Read the model definition and answer for the solid it produces. Units are mm, in the model's axes. A direction names the side the tool comes from. Give positions to 0.01 mm unless a question says otherwise; leave off trailing zeros. Loops run counter-clockwise (first coordinate to the right, second up) from the corner with the lowest first, then second, coordinate; pieces in that order, holes last. Notation, with made-up numbers: (70.25, 10.5) -> (122.25, 10.5) arc R18 ccw to (122.25, 26.5) -> close; hole circle Ø3 at (-7.75, 84). An arc over 180 degrees is marked (long way). Answer as CSV lines item,"result". Start each with the question number.
```python
from build123d import *

# Parameters (mm, degrees)
F0_R      = 2
F1_DEPTH  = 8
F3_DEPTH  = 185
F5_DEPTH  = 5
F6_R      = 2.5
F7_DEPTH  = 5
F8_R      = 2.012254
F9_DEPTH  = 3
F10_R     = 4
F10_R_2   = 2
F11_DEPTH = 4
F13_DEPTH = 340
F15_DEPTH = 320
F16_R     = 1.5
F17_DEPTH = 25


with BuildPart() as f1:
    # F0 (on Top) → F1 (new body)
    with BuildSketch(Plane.XY):
        Polygon((248.954639, 211.431908), (-84.845372, 211.431908), (-84.845372, -69.567305), (248.954639, -69.567305), (248.954639, -32.408092), align=None)
        with Locations((-44.415361, -24.153092)):
            Circle(F0_R, mode=Mode.SUBTRACT)
        with BuildLine():
            Line((-54.415363, 33.177276), (-54.415363, -42.732489))
            ThreePointArc((-54.415363, -42.732489), (-60.347495, -48.664621), (-66.279627, -42.732489))
            Line((-66.279627, -42.732489), (-66.279627, 33.177276))
            ThreePointArc((-66.279627, 33.177276), (-60.347495, 39.109408), (-54.415363, 33.177276))
        make_face(mode=Mode.SUBTRACT)
        with BuildLine():
            Line((-19.355729, -34.152674), (54.985007, -34.152674))
            ThreePointArc((54.985007, -34.152674), (63.564824, -42.732488), (54.98501, -51.312305))
            Line((54.98501, -51.312305), (-19.355726, -51.312305))
            ThreePointArc((-19.355726, -51.312305), (-27.935546, -42.732491), (-19.355729, -34.152674))
        make_face(mode=Mode.SUBTRACT)
        with Locations((80.044639, -24.153092)):
            Circle(F0_R, mode=Mode.SUBTRACT)
        with Locations((-44.415361, 48.236908)):
            Circle(F0_R, mode=Mode.SUBTRACT)
        with BuildLine():
            ThreePointArc((-34.415361, 23.177276), (-30.004497, 33.826044), (-19.355729, 38.236908))
            Line((-19.355729, 38.236908), (54.985007, 38.236908))
            ThreePointArc((54.985007, 38.236908), (65.633775, 33.826044), (70.044639, 23.177276))
            Line((70.044639, 23.177276), (70.044639, 0.90654))
            ThreePointArc((70.044639, 0.90654), (65.633775, -9.742228), (54.985007, -14.153092))
            Line((54.985007, -14.153092), (-19.355729, -14.153092))
            ThreePointArc((-19.355729, -14.153092), (-30.004497, -9.742228), (-34.415361, 0.90654))
            Line((-34.415361, 0.90654), (-34.415361, 23.177276))
        make_face(mode=Mode.SUBTRACT)
        with Locations((80.044639, 48.236908)):
            Circle(F0_R, mode=Mode.SUBTRACT)
        with BuildLine():
            ThreePointArc((212.465007, -34.152674), (221.044824, -42.732488), (212.46501, -51.312305))
            Line((212.46501, -51.312305), (105.104274, -51.312305))
            ThreePointArc((105.104274, -51.312305), (96.524457, -42.732491), (105.104271, -34.152674))
            Line((105.104271, -34.152674), (212.465007, -34.152674))
        make_face(mode=Mode.SUBTRACT)
        with Locations((237.524639, -24.153092)):
            Circle(F0_R, mode=Mode.SUBTRACT)
        with BuildLine():
            Line((90.044639, 0.90654), (90.044639, 23.177276))
            ThreePointArc((90.044639, 23.177276), (94.455503, 33.826044), (105.104271, 38.236908))
            Line((105.104271, 38.236908), (212.465007, 38.236908))
            ThreePointArc((212.465007, 38.236908), (223.113775, 33.826044), (227.524639, 23.177276))
            Line((227.524639, 23.177276), (227.524639, 0.90654))
            ThreePointArc((227.524639, 0.90654), (223.113775, -9.742228), (212.465007, -14.153092))
            Line((212.465007, -14.153092), (105.104271, -14.153092))
            ThreePointArc((105.104271, -14.153092), (94.455503, -9.742228), (90.044639, 0.90654))
        make_face(mode=Mode.SUBTRACT)
        with Locations((237.524639, 48.236908)):
            Circle(F0_R, mode=Mode.SUBTRACT)
        with BuildLine():
            Line((-54.415363, 180.316908), (-54.415363, 63.29654))
            ThreePointArc((-54.415363, 63.29654), (-60.347495, 57.364408), (-66.279627, 63.29654))
            Line((-66.279627, 63.29654), (-66.279627, 180.316908))
            ThreePointArc((-66.279627, 180.316908), (-60.347495, 186.24904), (-54.415363, 180.316908))
        make_face(mode=Mode.SUBTRACT)
        with BuildLine():
            Line((-34.415361, 73.29654), (-34.415361, 178.117276))
            ThreePointArc((-34.415361, 178.117276), (-30.004497, 188.766044), (-19.355729, 193.176908))
            Line((-19.355729, 193.176908), (54.985007, 193.176908))
            ThreePointArc((54.985007, 193.176908), (65.633775, 188.766044), (70.044639, 178.117276))
            Line((70.044639, 178.117276), (70.044639, 73.29654))
            ThreePointArc((70.044639, 73.29654), (65.633775, 62.647772), (54.985007, 58.236908))
            Line((54.985007, 58.236908), (-19.355729, 58.236908))
            ThreePointArc((-19.355729, 58.236908), (-30.004497, 62.647772), (-34.415361, 73.29654))
        make_face(mode=Mode.SUBTRACT)
        with Locations((-44.415361, 203.176908)):
            Circle(F0_R, mode=Mode.SUBTRACT)
        with Locations((80.044639, 203.176908)):
            Circle(F0_R, mode=Mode.SUBTRACT)
        with BuildLine():
            ThreePointArc((227.524639, 73.29654), (223.113775, 62.647772), (212.465007, 58.236908))
            Line((212.465007, 58.236908), (105.104271, 58.236908))
            ThreePointArc((105.104271, 58.236908), (94.455503, 62.647772), (90.044639, 73.29654))
            Line((90.044639, 73.29654), (90.044639, 178.117276))
            ThreePointArc((90.044639, 178.117276), (94.455503, 188.766044), (105.104271, 193.176908))
            Line((105.104271, 193.176908), (212.465007, 193.176908))
            Line((212.465007, 193.176908), (212.465007, 170.316908))
            ThreePointArc((212.465007, 170.316908), (223.113775, 165.906044), (227.524639, 155.257276))
            Line((227.524639, 155.257276), (227.524639, 73.29654))
        make_face(mode=Mode.SUBTRACT)
        with Locations((237.524639, 180.316908)):
            Circle(F0_R, mode=Mode.SUBTRACT)
    extrude(amount=F1_DEPTH)

    # F2 (on face) → F3 (join)
    with BuildSketch(Plane.XY.offset(8)):
        Polygon((15.154628, 211.431908), (-84.845372, 211.431908), (-84.845372, 71.431908), (-81.845372, 71.431908), (-81.845372, 208.431908), (15.154628, 208.431908), align=None)
    extrude(amount=F3_DEPTH)

    # F4 (on face) → F5 (cut)
    with BuildSketch(Plane(origin=(-84.845372, 0, 0), x_dir=(0, -1, 0), z_dir=(-1, 0, 0))):
        Polygon((-169.016169, 40), (-201.431908, 143.553324), (-201.431908, 40), align=None)
        Polygon((-71.431908, 193), (-206.431908, 193), (-158.537665, 40), (-71.431908, 40), align=None)
    extrude(amount=-F5_DEPTH, mode=Mode.SUBTRACT)

    # F6 (on face) → F7 (cut)
    with BuildSketch(Plane(origin=(0, 211.431908, 0), x_dir=(-1, 0, 0), z_dir=(0, 1, 0))):
        Polygon((12.845372, 83.034229), (12.845372, 55.132884), (75.345372, 55.132884), (75.345372, 148.132884), (67.845372, 148.132884), (67.845372, 178.132884), (2.845372, 178.132884), (1.345372, 83.215967), align=None)
        with Locations((11.345372, 185.632884)):
            Circle(F6_R)
        with Locations((1.345372, 185.632884)):
            Circle(F6_R)
        with Locations((75.345372, 161.632884)):
            Circle(F6_R)
        with Locations((75.345372, 185.632884)):
            Circle(F6_R)
        with Locations((75.345372, 47.632884)):
            Circle(F6_R)
        with Locations((65.345372, 47.632884)):
            Circle(F6_R)
        with Locations((1.345372, 47.632884)):
            Circle(F6_R)
        with Locations((1.345372, 71.632884)):
            Circle(F6_R)
    extrude(amount=-F7_DEPTH, mode=Mode.SUBTRACT)

    # F8 (on face) → F9 (join)
    with BuildSketch(Plane.XY.offset(40)):
        Polygon((14.154628, 208.488166), (-81.845372, 208.488166), (-81.845372, 201.431908), (-81.845372, 169.016169), (-81.845372, 71.523808), align=None)
        Polygon((-71.845372, 103.213636), (-71.845372, 198.488166), (-5.066284, 198.488166), align=None, mode=Mode.SUBTRACT)
        with Locations((-44.408604, 203.142822)):
            Circle(F8_R, mode=Mode.SUBTRACT)
    extrude(amount=-F9_DEPTH)

    # F10 (on face) → F11 (join)
    with BuildSketch(Plane.XY.offset(8)):
        with Locations((237.524639, 48.236908)):
            Circle(F10_R)
        with Locations((237.524639, 48.236908)):
            Circle(F10_R_2, mode=Mode.SUBTRACT)
        with Locations((237.524639, -24.153092)):
            Circle(F10_R)
        with Locations((237.524639, -24.153092)):
            Circle(F10_R_2, mode=Mode.SUBTRACT)
        with Locations((80.044639, 48.236908)):
            Circle(F10_R)
        with Locations((80.044639, 48.236908)):
            Circle(F10_R_2, mode=Mode.SUBTRACT)
        with Locations((80.044639, -24.153092)):
            Circle(F10_R)
        with Locations((80.044639, -24.153092)):
            Circle(F10_R_2, mode=Mode.SUBTRACT)
    extrude(amount=F11_DEPTH)

    # F12 (on face) → F13 (cut)
    with BuildSketch(Plane.YZ.offset(248.954639)):
        Polygon((57.743425, 4), (37.743425, 4), (37.743425, 0), (211.431908, 0), (211.431908, 8), (57.743425, 8), align=None)
    extrude(amount=-F13_DEPTH, mode=Mode.SUBTRACT)

    # F14 (on face) → F15 (cut)
    with BuildSketch(Plane(origin=(0, 211.431908, 0), x_dir=(-1, 0, 0), z_dir=(0, 1, 0))):
        Polygon((-69.711687, 8), (-69.711687, 4), (-89.711687, 4), (-89.711687, 0), (-20.75227, 0), (93.97424, 0), (93.97424, 17.639369), (93.97424, 194.899216), (-20.75227, 194.899216), (-20.75227, 10.883192), align=None)
    extrude(amount=-F15_DEPTH, mode=Mode.SUBTRACT)

    # F16 (on face) → F17 (cut)
    with BuildSketch(Plane.XY.offset(8)):
        with Locations((214.26287, -63.217305)):
            Circle(F16_R)
        with Locations((112.66287, -63.217305)):
            Circle(F16_R)
        with Locations((172.65287, -63.217305)):
            Circle(F16_R)
    extrude(amount=-F17_DEPTH, mode=Mode.SUBTRACT)


solid = f1.part
```
(1) Each of these flat-tipped pins is pushed along its axis until it touches: P1, Ø6, axis at x = 229.5, y = -37, coming from the +Z side; P2, Ø1.2, axis at x = 228, z = 1.5, coming from the +Y side; P3, Ø4.5, axis at y = -17.5, z = 1.5, coming from the -X side. Where does it stop, or does it pass through?
(2) Find section D-D on x = 223. Write down the section's boundary in (y, z), then the cut area to 3 significant figures.
(3) Find the intervals of material crossed by line 1 along Y through (x, z) = (129, 5.25); line 2 along X through (y, z) = (21, 3.5); line 3 along X through (y, z) = (-63.5, 5.5), in increasing order. Write a range as from..to.
(4) Find section B-B on x = 194. Write down the section's boundary in (y, z), then the cut area to 3 significant figures.
(5) The mould has two halves that part along Y. Classify faces 4 (the face through (239.2, 46.5, 12)), 5 (the face through (235.527, 48.325, 7.944)): pulls with the +Y half, pulls with the -Y half, needs draft (parallel to the pull), parting line crosses it, or undercut.
(6) Find section C-C on z = 2. Write down the section's boundary in (x, y) (3 decimals), then the cut area to 3 significant figures.
(7) A tool of negligible diameter and unlimited length cuts with its end or side. For faces 1 (the face through (94.34, 33.71, 3.94)), 2 (the face through (238, -22, 12)), 3 (the face through (241.34, 49.44, 9.97)), from which of +Z, -Z, +X, -X, +Y, -Y can it reach the whole face along a straight path? Write none if from no direction.
(8) Find section A-A on y = 21. Write down the section's boundary in (x, z).
Answer block:
1,P1,"stops at z = 8"
1,P2,"stops at y = 37.74"
1,P3,"stops at x = 89.71"
2,outline,"(-69.57, 0) -> (-9.85, 0) -> (-9.85, 8) -> (-69.57, 8) -> close; (33.94, 0) -> (37.74, 0) -> (37.74, 4) -> (57.74, 4) -> (57.74, 8) -> (33.94, 8) -> close"
2,area,"588 mm2"
3,line 1,"y = -69.57..-51.31, -34.15..-14.15, 38.24..57.74"
3,line 2,"x = 89.71..90.04, 227.52..248.95"
3,line 3,"x = 69.71..111.19, 114.14..171.18, 174.13..212.79, 215.74..248.95"
4,outline,"(-69.57, 0) -> (-51.31, 0) -> (-51.31, 8) -> (-69.57, 8) -> close; (-34.15, 0) -> (-14.15, 0) -> (-14.15, 8) -> (-34.15, 8) -> close; (38.24, 4) -> (57.74, 4) -> (57.74, 8) -> (38.24, 8) -> close"
4,area,"384 mm2"
5,face 4,"needs draft"
5,face 5,"undercut"
6,outline,"(89.712, -69.567) -> (248.955, -69.567) -> (248.955, 37.743) -> (216.289, 37.743) arc R15.06 cw to (227.525, 23.177) -> (227.525, 0.907) arc R15.06 cw to (212.465, -14.153) -> (105.104, -14.153) arc R15.06 cw to (90.045, 0.907) -> (90.045, 23.177) arc R15.06 cw to (101.281, 37.743) -> (89.712, 37.743) -> close; hole (105.104, -51.312) -> (212.465, -51.312) arc R8.58 ccw to (212.465, -34.153) -> (105.104, -34.153) arc R8.58 ccw to start; hole circle Ø3 at (112.663, -63.217); hole circle Ø3 at (172.653, -63.217); hole circle Ø3 at (214.263, -63.217); hole circle Ø4 at (237.525, -24.153)"
6,area,"8,030 mm2"
7,face 1,"+Z, -Z"
7,face 2,"+Z, +X, -X, +Y, -Y"
7,face 3,"+Z"
8,outline,"(70.04, 4) -> (89.71, 4) -> (89.71, 0) -> (90.04, 0) -> (90.04, 8) -> (70.04, 8) -> close; (227.52, 0) -> (248.95, 0) -> (248.95, 8) -> (227.52, 8) -> close"
